The listing builds one solid part. Answer for the finished solid, in the listing's coordinates (mm). Face numbers are marked on the shaded views. A direction names the side the tool comes from. Round coordinates to 2 decimals unless told otherwise and drop trailing zeros. Write each loop counter-clockwise with the first axis right and the second up, starting at its lowest first coordinate (ties: lowest second). Pieces come first, ordered by that corner, then holes. Notation, with made-up numbers: (24, 29) - (64, 29) arc R18 cw to (64, 57) - close; hole circle Ø3 at (15, 52.25). An arc over 180 degrees is marked (long way). Answer as CSV lines item,"result". Start each with the question number.
Item 1: A cutting plane is placed at D-D on x = 36. Determine the outline of the cut face in (y, z).
Item 2: A cutting plane is placed at B-B on z = 5.5. Determine the outline of the cut face in (x, y), and give its area (3 significant figures).
Item 3: Straight lines are drawn through the part: line 1 along Y through (x, z) = (48, 2.9); line 2 along X through (y, z) = (17, 2.1); line 3 along X through (y, z) = (18, 1.5). For each, find the intervals that lie inside material, in ascending order. Write a range as [from, to].
Item 4: A cutting plane is placed at C-C on z = 3. Determine the outline of the cut face in (x, y).
Item 5: A flat-ended cylindrical pin translates along its axis: pin 1 (5.5 mm diameter, centred on x = 4, y = 17, fed in from +Z). Find the tip coordinate at first contact, or state that the pin passes through.
Item 6: A cutting plane is placed at A-A on y = 4. Determine the outline of the cut face in (x, z), and give its area (3 significant figures).
Item 7: Which of the six approach directions +Z, -Z, +X, -X, +Y, -Y give full straight-line access (tool end or side, diameter ignored) to the marked faces 1, 2 and 3?
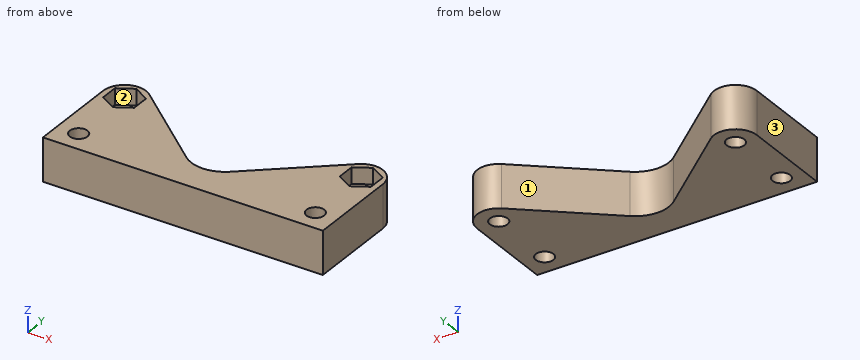
```python
from build123d import *

# Parameters (mm, degrees)
SKETCH1_R           = 1.65
BOSS_EXTRUDE1_DEPTH = 8
CUT_EXTRUDE1_DEPTH  = 3


with BuildPart() as part:
    # Sketch1 → Boss-Extrude1 (new body)
    with BuildSketch(Plane.XY):
        with BuildLine():
            Line((0, 0), (52, 0))
            Line((52, 0), (52, 17))
            ThreePointArc((52, 17), (49.689734101, 20.625575633), (45.427600665, 20.06312939))
            Line((45.427600665, 20.06312939), (30.036241487, 7.137550003))
            ThreePointArc((30.036241487, 7.137550003), (26, 5.667546504), (21.963758513, 7.137550003))
            Line((21.963758513, 7.137550003), (6.572399335, 20.06312939))
            ThreePointArc((6.572399335, 20.06312939), (2.310265899, 20.625575633), (0, 17))
            Line((0, 17), (0, 0))
        make_face()
        with Locations((4, 17)):
            Circle(SKETCH1_R, mode=Mode.SUBTRACT)
        with Locations((48, 17)):
            Circle(SKETCH1_R, mode=Mode.SUBTRACT)
        with Locations((4, 4)):
            Circle(SKETCH1_R, mode=Mode.SUBTRACT)
        with Locations((48, 4)):
            Circle(SKETCH1_R, mode=Mode.SUBTRACT)
    extrude(amount=BOSS_EXTRUDE1_DEPTH)

    # Sketch2 → Cut-Extrude1 (cut)
    with BuildSketch(Plane.XY.offset(8)):
        Polygon((4, 13.651368439), (6.9, 15.325684219), (6.9, 18.674315781), (4, 20.348631561), (1.1, 18.674315781), (1.1, 15.325684219), align=None)
        Polygon((48, 13.651368439), (50.9, 15.325684219), (50.9, 18.674315781), (48, 20.348631561), (45.1, 18.674315781), (45.1, 15.325684219), align=None)
    extrude(amount=-CUT_EXTRUDE1_DEPTH, mode=Mode.SUBTRACT)


solid = part.part
```
Geometry says:
1,outline,"(0, 0) - (12.15, 0) - (12.15, 8) - (0, 8) - close"
2,outline,"(0, 0) - (52, 0) - (52, 17) arc R4 ccw to (45.43, 20.06) - (30.04, 7.14) arc R6.28 cw to (21.96, 7.14) - (6.57, 20.06) arc R4 ccw to (0, 17) - close; hole (1.1, 15.33) - (4, 13.65) - (6.9, 15.33) - (6.9, 18.67) - (4, 20.35) - (1.1, 18.67) - close; hole circle Ø3.3 at (4, 4); hole (45.1, 15.33) - (48, 13.65) - (50.9, 15.33) - (50.9, 18.67) - (48, 20.35) - (45.1, 18.67) - close; hole circle Ø3.3 at (48, 4)"
2,area,"660 mm^2"
3,line 1,"y = [0, 2.35], [5.65, 15.35], [18.65, 21]"
3,line 2,"x = [0, 2.35], [5.65, 10.22], [41.78, 46.35], [49.65, 52]"
3,line 3,"x = [0.13, 2.69], [5.31, 9.03], [42.97, 46.69], [49.31, 51.87]"
4,outline,"(0, 0) - (52, 0) - (52, 17) arc R4 ccw to (45.43, 20.06) - (30.04, 7.14) arc R6.28 cw to (21.96, 7.14) - (6.57, 20.06) arc R4 ccw to (0, 17) - close; hole circle Ø3.3 at (4, 4); hole circle Ø3.3 at (4, 17); hole circle Ø3.3 at (48, 4); hole circle Ø3.3 at (48, 17)"
5,pin 1,"stops at z = 5"
6,outline,"(0, 0) - (2.35, 0) - (2.35, 8) - (0, 8) - close; (5.65, 0) - (46.35, 0) - (46.35, 8) - (5.65, 8) - close; (49.65, 0) - (52, 0) - (52, 8) - (49.65, 8) - close"
6,area,"363 mm^2"
7,face 1,"+Z, -Z, +Y"
7,face 2,"+Z"
7,face 3,"+Z, -Z, -X, +Y, -Y"
